```python
from build123d import *

# Parameters (mm, degrees)
SKETCH1_W           = 2
SKETCH1_H           = 100
BOSS_EXTRUDE1_DEPTH = 58
BOSS_EXTRUDE2_DEPTH = 2


with BuildPart() as part:
    # Sketch1 → Boss-Extrude1 (new body)
    with BuildSketch(Plane.XY):
        with Locations((-0.084337349, -26.626506024)):
            Rectangle(SKETCH1_W, SKETCH1_H)
    extrude(amount=BOSS_EXTRUDE1_DEPTH)

    # Sketch2 → Boss-Extrude2 (add)
    with BuildSketch(Plane.XZ.offset(76.626506024)):
        with BuildLine():
            Line((0.915662651, 58), (-1.084337349, 58))
            Line((-1.084337349, 58), (-1.084337349, 0))
            Line((-1.084337349, 0), (105.357714941, 0))
            add(Edge.make_bspline(
                [(0.915662651, 58), (63.617404925, 50.187924703), (105.357714941, 0)],
                knots=[0, 0, 0, 1, 1, 1], degree=2))
        make_face()
    extrude(amount=-BOSS_EXTRUDE2_DEPTH)


solid = part.part
```
Part model, mm, in its own coordinate system. A direction names the side the tool comes from. Give positions to 0.01 mm unless a question says otherwise; leave off trailing zeros. Write each loop counter-clockwise with the first axis right and the second up, starting at its lowest first coordinate (ties: lowest second). Pieces come first, ordered by that corner, then holes. Notation, with made-up numbers: (11.25, -25) -> (39.25, -25) arc R16 cw to (39.25, -1) -> close; hole circle Ø3 at (69.5, 82.25). An arc over 180 degrees is marked (long way). Put each result on its own line as item: value. Start each with the question number.
Item 1: Pin check, flat tips, straight feed: pin 1 Ø4 at (x, z) = (81, 24.5) entering from +Y; pin 2 Ø12 at (y, z) = (-64.5, 7.5) entering from +X; pin 3 Ø12 at (x, z) = (88.5, 30) entering from -Y. Stop position of each tip, or through.
Item 2: Wall check: L1, parallel to X at y = 16.5, z = 6.5; L2, parallel to Y at x = 3, z = 42.5. Give the ranges that are in metal, low to high. Write a range as [from, to].
Item 3: Cut at A-A (y = -5). List the corners of the cut face in (x, z), then the cut area to 3 significant figures.
Item 4: Which spindle directions (+Z, -Z, +X, -X, +Y, -Y) get a long thin tool onto all of the face, cutting with end or side? Do faces 1 (the face through (0.6, -26.4, 0)), 2 (the face through (41, -74.627, 23)). Say none if no direction does.
Answer list:
1. pin 1: stops at y = -74.63
1. pin 2: stops at x = 0.92
1. pin 3: passes through
2. L1: x = [-1.08, 0.92]
2. L2: y = [-76.63, -74.63]
3. outline: (-1.08, 0) -> (0.92, 0) -> (0.92, 58) -> (-1.08, 58) -> close
3. area: 116 mm2
4. face 1: -Z, +X, -X, +Y, -Y
4. face 2: +Z, -Z, +X, +Y
